The model under review builds one solid part; all positions refer to its coordinate system, in mm. Give positions to 0.01 mm unless a question says otherwise; leave off trailing zeros. Loops run counter-clockwise (first coordinate to the right, second up) from the corner with the lowest first, then second, coordinate; pieces in that order, holes last. Notation, with made-up numbers: M -22,3 L 29,3 A25 cw 29,24 Z; hole C 71.25,-35 d1. An arc over 180 degrees is marked long. Put each result on its own line as item: value. Start each with the question number.
```python
from build123d import *

# Parameters (mm, degrees)
SKETCH_1_R      = 1.5
EXTRUDE_1_DEPTH = 3
FILLET_1_R      = 2


with BuildPart() as part:
    # Эскиз1 → Бобышка-Вытянуть1 (new body)
    with BuildSketch(Plane(origin=(0, 0, 0), x_dir=(1, 0, 0), z_dir=(0, 1, 0))):
        with BuildLine():
            Line((-3.863363367, 13.30042486), (-8.639745084, 4.930152864))
            ThreePointArc((-8.639745084, 4.930152864), (-9.947442002, 0), (-8.639745084, -4.930152864))
            Line((-8.639745084, -4.930152864), (-3.47415751, -13.982480667))
            ThreePointArc((-3.47415751, -13.982480667), (0, -16), (3.47415751, -13.982480667))
            Line((3.47415751, -13.982480667), (8.639745084, -4.930152864))
            ThreePointArc((8.639745084, -4.930152864), (9.947442002, 0), (8.639745084, 4.930152864))
            Line((8.639745084, 4.930152864), (3.863363367, 13.30042486))
            Line((3.863363367, 13.30042486), (3.47415751, 13.982480667))
            ThreePointArc((3.47415751, 13.982480667), (0, 16), (-3.47415751, 13.982480667))
            Line((-3.47415751, 13.982480667), (-3.863363367, 13.30042486))
        make_face()
        with Locations((0, 12)):
            Circle(SKETCH_1_R, mode=Mode.SUBTRACT)
        with Locations((0, -12)):
            Circle(SKETCH_1_R, mode=Mode.SUBTRACT)
    extrude(amount=EXTRUDE_1_DEPTH)

    # Скругление1
    fillet_1_edges = [part.edges().sort_by_distance(p)[0] for p in [
        (0, 3, 16),
        (6.056951297, 3, 9.456316766),
        (9.947442002, 3, 0),
        (6.056951297, 3, -9.456316766),
        (0, 3, -16),
        (-6.056951297, 3, -9.456316766),
        (-9.947442002, 3, 0),
        (-6.056951297, 3, 9.456316766),
    ]]
    fillet(fillet_1_edges, radius=FILLET_1_R)


solid = part.part
```
Item 1: Draft analysis for pull direction Z (two halves, no side actions). For faces 1 (the cylindrical face through (9.947, 0.493, 0.072)), 2 (the cylindrical face through (-0.325, 1.479, -10.536)), 3 (the cylindrical face through (-0.325, 1.479, 13.464)), 4 (the cylindrical face through (5.6, 2.4, 9.1)), state which applies: +Z half, -Z half, draft (parallel to the pull), parting line (faces both ways), or undercut.
Item 2: To check wall thickness, follow L1, parallel to Z at x = 1.25, y = 2.2; L2, parallel to X at y = 1.8, z = -12; L3, parallel to X at y = 2.75, z = -13. State the ranges of each line that lie inside material, in increasing order. Write a range as [from, to].
Item 3: Consider section B-B, the plane x = 0. Give the number of separate pieces and of enclosed holes in the cut face, plus the area to 3 significant figures.
Item 4: Clearance check with flat-ended pins moving along their axes: pin 1 Ø1.5 at (y, z) = (1.5, -4) entering from -X; pin 2 Ø2.5 at (x, z) = (0, -12) entering from -Y. State where each tip first meets the part, or that it passes through.
Item 5: Consider section A-A, the plane y = 0.4. Write out the cut boundary in (x, z), plus the area to 3 significant figures.
Report:
1. face 1: parting line
1. face 2: undercut
1. face 3: undercut
1. face 4: +Z half
2. L1: [-15.38, -12.83], [-11.17, 11.17], [12.83, 15.38]
2. L2: [-4.41, -1.5], [1.5, 4.41]
2. L3: [-2.85, -1.12], [1.12, 2.85]
3. separate pieces: 3
3. enclosed holes: 0
3. area: 76.3 mm²
4. pin 1: x = -9.37
4. pin 2: through
5. outline: M -8.64,-4.93 L -3.47,-13.98 A4 ccw 3.47,-13.98 L 8.64,-4.93 A9.95 ccw 8.64,4.93 L 3.47,13.98 A4 ccw -3.47,13.98 L -8.64,4.93 A9.95 ccw Z; hole C 0,-12 d3; hole C 0,12 d3
5. area: 413 mm²
